Check sheet for the modelled part. Datum: model origin and axes. Units: mm. Face numbers are marked on the shaded views. A direction names the side the tool comes from. Coordinates: 2 decimals unless noted, no trailing zeros. Loops run counter-clockwise (first coordinate to the right, second up) from the corner with the lowest first, then second, coordinate; pieces in that order, holes last. Notation, with made-up numbers: (58, -7) -> (75, -7) arc R20 cw to (75, 15) -> close; hole circle Ø4 at (28, 26.5). An arc over 180 degrees is marked (long way). Use CSV: the item, a comma, the result in double quotes. Start each with the question number.
1. Release check for a two-part mould opening along Z. For the marked faces 1, 2 and 3 record: pulls with the +Z half, pulls with the -Z half, needs draft (parallel to the pull), parting line crosses it, or undercut.
2. Sectioned sample at C-C, the plane z = 17.5. Record the cut outline in (x, y).
3. Set-up check for the marked faces 4, 5 and 6: record each of +Z, -Z, +X, -X, +Y, -Y from which the full face is reachable in a straight line by a thin tool's end or side.
4. Gauge pin test, flat ends, axial feed: pin 1 (1 mm diameter, centred on y = 11, z = 16, fed in from -X); pin 2 (10 mm diameter, centred on y = -7.5, z = 16, fed in from -X); pin 3 (6 mm diameter, centred on x = -2, z = 20, fed in from +Y). Record the tip position at first contact, or that the pin passes through.
5. Sectioned sample at D-D, the plane z = 10.75. Record the cut outline in (x, y).
6. Sectioned sample at B-B, the plane z = 4.75. Record the cut outline in (x, y).
7. Thickness scan on L1, parallel to Y at x = 0, z = 15.5; L2, parallel to Y at x = 0, z = 7.25; L3, parallel to X at y = -3.25, z = 18.5. Record the ranges inside material, lowest first.
Autodesk Inventor part; units mm, degrees
ref_plane "YZ Plane" through (0, 0, 0) normal (1, 0, 0) x (0, 1, 0)
ref_plane "XZ Plane" through (0, 0, 0) normal (0, 1, 0) x (-1, 0, 0)
ref_plane "XY Plane" through (0, 0, 0) normal (0, 0, 1) x (1, 0, 0)
sketch "草图1" plane through (0, 0, 0) normal (0, 0, 1) x (1, 0, 0)
  line L0 (8.0829, 14) -> (16.1658, 0)
  line L1 (16.1658, 0) -> (8.0829, -14)
  line L2 (8.0829, -14) -> (-8.0829, -14)
  line L3 (-8.0829, -14) -> (-16.1658, 0)
  line L4 (-16.1658, 0) -> (-8.0829, 14)
  line L5 (-8.0829, 14) -> (8.0829, 14)
  point P0 (0, 0)
  point P1 (0, 0)
extrude "拉伸1" add sketch "草图1" along normal blind 9
sketch "草图2" plane through (0, 0, 9) normal (0, 0, 1) x (1, 0, 0)
  circle A0 centre (0, 0) radius 11.5
  dimension "d4" = 23
extrude "拉伸2" add sketch "草图2" along normal blind 3
sketch "草图3" plane through (0, 0, 12) normal (0, 0, 1) x (1, 0, 0)
  circle A0 centre (0, 0) radius 13.5
  dimension "d7" = 27
extrude "拉伸3" add sketch "草图3" along normal blind 12
chamfer "倒角1" distance 2 angle 45 2 edges at (-13.5, 0, 24) (-13.5, 0, 12)
sketch "草图4" plane through (0, 0, 24) normal (0, 0, 1) x (1, 0, 0)
  circle A0 centre (0, 0) radius 11.5
hole "孔1" at (0, 0, 24) direction (0, 0, -1) diameter 11 end through all
thread "螺纹1"
chamfer "倒角2" distance 1 angle 45 6 edges at (12.1244, -7, 0) (12.1244, 7, 0) (0, 14, 0) (-12.1244, 7, 0) (0, -14, 0) (-12.1244, -7, 0)
properties part number "3-锁紧螺母" material "灰口铁"
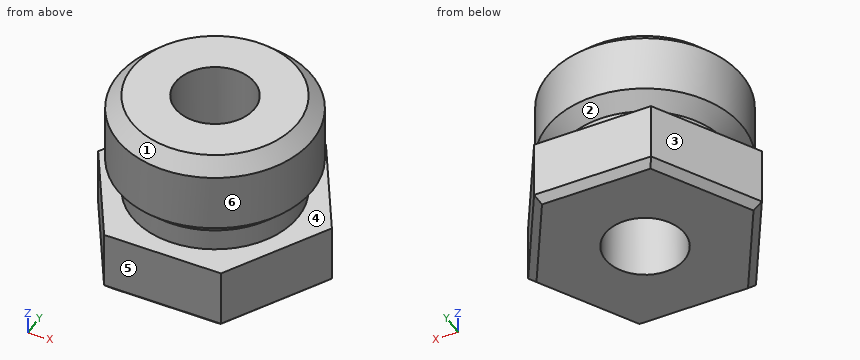
Completed:
1,face 1,"pulls with the +Z half"
1,face 2,"undercut"
1,face 3,"needs draft"
2,outline,"circle Ø27 at (0, 0); hole circle Ø11 at (0, 0)"
3,face 4,"none"
3,face 5,"+Z, -Z, +X, -X, -Y"
3,face 6,"+Z"
4,pin 1,"x = -8.49"
4,pin 2,"x = -13.27"
4,pin 3,"y = 13.5"
5,outline,"circle Ø23 at (0, 0); hole circle Ø11 at (0, 0)"
6,outline,"(-16.17, 0) -> (-8.08, -14) -> (8.08, -14) -> (16.17, 0) -> (8.08, 14) -> (-8.08, 14) -> close; hole circle Ø11 at (0, 0)"
7,L1,"-13.5 to -5.5, 5.5 to 13.5"
7,L2,"-14 to -5.5, 5.5 to 14"
7,L3,"-13.1 to -4.44, 4.44 to 13.1"
